Input: part model. Units: mm. Frame: model coordinates. Face numbers are marked on the shaded views. A direction names the side the tool comes from. Round coordinates to 2 decimals unless told otherwise and drop trailing zeros. Loops run counter-clockwise (first coordinate to the right, second up) from the corner with the lowest first, then second, coordinate; pieces in that order, holes last. Notation, with made-up numbers: (37, 69) - (89, 69) arc R19 ccw to (89, 104) - close; hole circle Ø9 at (-39.5, -39). An arc over 180 degrees is marked (long way). Write each question's results on one line, items separated by ' | '.
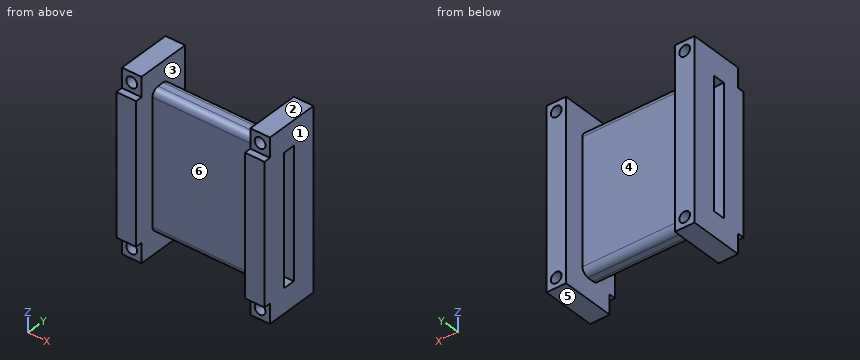
from build123d import *

# Parameters (mm, degrees)
SKETCH1_W           = 40.9
SKETCH1_H           = 5.9
SKETCH1_W_2         = 38.5
SKETCH1_H_2         = 3.5
BOSS_EXTRUDE1_DEPTH = 32.25
FILLET2_R           = 2
SKETCH2_W           = 53
SKETCH2_H           = 18
SKETCH2_W_2         = 38.5
SKETCH2_H_2         = 3.5
BOSS_EXTRUDE2_DEPTH = 5.8
SKETCH3_W           = 53
SKETCH3_H           = 18
SKETCH3_W_2         = 38.5
SKETCH3_H_2         = 3.5
BOSS_EXTRUDE3_DEPTH = 5.8
SKETCH4_R           = 1.6
CUT_EXTRUDE1_DEPTH  = 64.056363676
SKETCH15_W          = 38.5
SKETCH15_H          = 3.5
SKETCH15_W_2        = 5.8
SKETCH15_H_2        = 2
CUT_EXTRUDE5_DEPTH  = 66.344682263


with BuildPart() as part:
    # Sketch1 → Boss-Extrude1 (new body)
    with BuildSketch(Plane(origin=(0, 0, 0), x_dir=(0, 0, -1), z_dir=(1, 0, 0))):
        with Locations((20.45, 2.95)):
            Rectangle(SKETCH1_W, SKETCH1_H)
        with Locations((20.45, 2.95)):
            Rectangle(SKETCH1_W_2, SKETCH1_H_2, mode=Mode.SUBTRACT)
    extrude(amount=BOSS_EXTRUDE1_DEPTH)

    # Fillet2
    fillet2_edges = [part.edges().sort_by_distance(p)[0] for p in [
        (16.125, 5.9, 0),
        (16.125, 5.9, -40.9),
        (16.125, 0, -40.9),
        (16.125, 0, 0),
    ]]
    fillet(fillet2_edges, radius=FILLET2_R)

    # Sketch2 → Boss-Extrude2 (add)
    with BuildSketch(Plane(origin=(32.25, 0, 0), x_dir=(0, 0, -1), z_dir=(1, 0, 0))):
        with Locations((20.45, 2.95)):
            Rectangle(SKETCH2_W, SKETCH2_H)
        with Locations((20.45, 2.95)):
            Rectangle(SKETCH2_W_2, SKETCH2_H_2, mode=Mode.SUBTRACT)
    extrude(amount=BOSS_EXTRUDE2_DEPTH)

    # Sketch3 → Boss-Extrude3 (add)
    with BuildSketch(Plane.ZY):
        with Locations((-20.45, 2.95)):
            Rectangle(SKETCH3_W, SKETCH3_H)
        with Locations((-20.45, 2.95)):
            Rectangle(SKETCH3_W_2, SKETCH3_H_2, mode=Mode.SUBTRACT)
    extrude(amount=BOSS_EXTRUDE3_DEPTH)

    # Sketch4 → Cut-Extrude1 (cut, through all)
    with BuildSketch(Plane(origin=(0, 11.95, 0), x_dir=(1, 0, 0), z_dir=(0, 1, 0))):
        with Locations(Location((-2.9, 44.05, 0), (0, 0, 270))):
            Circle(SKETCH4_R)
        with Locations(Location((35.15, 44.05, 0), (0, 0, 270))):
            Circle(SKETCH4_R)
        with Locations(Location((-2.9, -3.15, 0), (0, 0, 270))):
            Circle(SKETCH4_R)
        with Locations(Location((35.15, -3.15, 0), (0, 0, 270))):
            Circle(SKETCH4_R)
    extrude(amount=-CUT_EXTRUDE1_DEPTH, mode=Mode.SUBTRACT)

    # Sketch15 → Cut-Extrude5 (cut, through all)
    with BuildSketch(Plane.ZY.offset(5.8)):
        with Locations((-20.45, 2.95)):
            Rectangle(SKETCH15_W, SKETCH15_H)
        with Locations((-44.05, -5.05)):
            Rectangle(SKETCH15_W_2, SKETCH15_H_2)
        with Locations((3.15, -5.05)):
            Rectangle(SKETCH15_W_2, SKETCH15_H_2)
    extrude(amount=-CUT_EXTRUDE5_DEPTH, mode=Mode.SUBTRACT)


solid = part.part
1. Section query D-D, the plane z = -30.5. Output: boundary loops of the cut face in (x, y).
Answer:
outline: (-5.8, -6.05) - (0, -6.05) - (0, 0) - (32.25, 0) - (32.25, -6.05) - (38.05, -6.05) - (38.05, 1.2) - (-5.8, 1.2) - close; (-5.8, 4.7) - (38.05, 4.7) - (38.05, 11.95) - (32.25, 11.95) - (32.25, 5.9) - (0, 5.9) - (0, 11.95) - (-5.8, 11.95) - close
2. Contact query for flat-ended pins moving along their axis: pin 1 (4.5 mm diameter, centred on x = -3.5, z = 3.5, fed in from -Y); pin 2 (6 mm diameter, centred on x = 12.5, z = -6.5, fed in from -Y); pin 3 (1 mm diameter, centred on x = 34.5, y = -5.5, fed in from -Z). Output: stop coordinate, or through.
Answer:
pin 1: y = -4.05 | pin 2: y = 0 | pin 3: z = -41.15
3. Mould query, pull axis X, two halves, no side actions, for the marked faces 1, 2 and 3. Classes: pulls with the +X half, pulls with the -X half, needs draft (parallel to the pull), parting line crosses it, or undercut.
Answer:
face 1: pulls with the +X half | face 2: needs draft | face 3: undercut
4. Section query C-C, the plane z = 3.15. Output: boundary loops of the cut face in (x, y).
Answer:
outline: (-5.8, -4.05) - (-4.5, -4.05) - (-4.5, 11.95) - (-5.8, 11.95) - close; (-1.3, -4.05) - (0, -4.05) - (0, 11.95) - (-1.3, 11.95) - close; (32.25, -4.05) - (33.55, -4.05) - (33.55, 11.95) - (32.25, 11.95) - close; (36.75, -4.05) - (38.05, -4.05) - (38.05, 11.95) - (36.75, 11.95) - close
5. Line query: line 1 (Z direction, x = 35, y = 5.5); line 2 (X direction, y = 3.5, z = -44.05); line 3 (X direction, y = -3.5, z = -12.5). Output: solid intervals per line, ascending. Write a range as [from, to].
Answer:
line 1: [-46.95, -45.64], [-42.46, 1.56], [4.74, 6.05] | line 2: [-5.8, -4.5], [-1.3, 0], [32.25, 33.55], [36.75, 38.05] | line 3: [-5.8, 0], [32.25, 38.05]
6. Section query B-B, the plane x = -2.9. Output: boundary loops of the cut face in (y, z).
Answer:
outline: (-6.05, -41.15) - (-4.05, -41.15) - (-4.05, -42.45) - (11.95, -42.45) - (11.95, 1.55) - (-4.05, 1.55) - (-4.05, 0.25) - (-6.05, 0.25) - close; (-4.05, -46.95) - (11.95, -46.95) - (11.95, -45.65) - (-4.05, -45.65) - close; (-4.05, 4.75) - (11.95, 4.75) - (11.95, 6.05) - (-4.05, 6.05) - close; hole (1.2, -39.7) - (4.7, -39.7) - (4.7, -1.2) - (1.2, -1.2) - close
7. Section query A-A, the plane y = 10.5. Output: boundary loops of the cut face in (x, z).
Answer:
outline: (-5.8, -46.95) - (0, -46.95) - (0, 6.05) - (-5.8, 6.05) - close; (32.25, -46.95) - (38.05, -46.95) - (38.05, 6.05) - (32.25, 6.05) - close; hole circle Ø3.2 at (-2.9, -44.05); hole circle Ø3.2 at (-2.9, 3.15); hole circle Ø3.2 at (35.15, -44.05); hole circle Ø3.2 at (35.15, 3.15)
8. Set-up query: the marked faces 4, 5 and 6. Return all of +Z, -Z, +X, -X, +Y, -Y with unobstructed straight access to the full face (end or side cutting, diameter ignored); none if empty.
Answer:
face 4: +Z, -Z, +Y | face 5: -Z, +X, -X, +Y, -Y | face 6: +Z, -Z, -Y
